For this review, take the finished solid that the model builds, in its own axes (mm). Coordinates: 2 decimals unless noted, no trailing zeros. Loops run counter-clockwise (first coordinate to the right, second up) from the corner with the lowest first, then second, coordinate; pieces in that order, holes last. Notation, with made-up numbers: (42.5, 89) -> (64.5, 89) arc R27 cw to (64.5, 115) -> close; hole circle Ø7 at (71.5, -28.75). An arc over 180 degrees is marked (long way). One line per item, written item: value.
Autodesk Inventor part; units mm, degrees
sketch "Эскиз1" plane through (0, 0, 0) normal (0, 1, 0) x (-1, 0, 0)
  line L0 (105, 10) -> (-105, 10)
  line L1 (-105, -10) -> (105, -10)
  line L2 (105, 10) -> (-105, -10) construction
  line L3 (-105, 10) -> (105, -10) construction
  arc A0 (-105, 10) -> (-105, -10) centre (-105, 0) ccw
  arc A1 (105, -10) -> (105, 10) centre (105, 0) ccw
  line L4 (0, -14) -> (0, 14) construction
  circle A2 centre (105, 0) radius 4
  circle A3 centre (-105, 0) radius 4
  circle A4 centre (0, 0) radius 4
  line L5 (-161, 0) -> (161, 0)
  point P0 (0, 10)
  point P1 (0, -10)
  dimension "d2" = 210
  dimension "d5" = 8
  dimension "d6" = 8
  dimension "d9" = 8
  dimension "d17" = 10
extrude "Выдавливание1" add sketch "Эскиз1" along normal mid plane 4 contours A1 L5 A2 A4 A3 A0 L0 | A1 L1 A0 L5 A3 A4 A2
properties part number "Рельс платформы подъёмника"
1. To check wall thickness, follow probe 1 along X at (y, z) = (-0.75, 0); probe 2 along Z at (x, y) = (105, -0.85); probe 3 along X at (y, z) = (-0.15, -2.75). State the ranges of each line that lie inside material, in increasing order. Write a range as from..to.
Return value:
probe 1: x = -115..-109, -101..-4, 4..101, 109..115
probe 2: z = -10..-4, 4..10
probe 3: x = -114.61..-107.9, -102.1..-2.9, 2.9..102.1, 107.9..114.61
2. Insertion check: pin 1 Ø7 at (x, z) = (-105, 0) entering from -Y; pin 2 Ø2 at (y, z) = (-0.5, 3) entering from +X; pin 3 Ø2 at (y, z) = (-0.5, -3.5) entering from -X. Each pin has a flat end and moves straight along its axis. Give the tip position at first contact, or say it passes through.
Return value:
pin 1: passes through
pin 2: stops at x = 114.8
pin 3: stops at x = -114.68
3. Take a section at A-A, the plane z = 0. Give the boundary of the cut face in (x, y), and give its area (3 significant figures).
Return value:
outline: (-115, -2) -> (-109, -2) -> (-109, 2) -> (-115, 2) -> close; (-101, -2) -> (-4, -2) -> (-4, 2) -> (-101, 2) -> close; (4, -2) -> (101, -2) -> (101, 2) -> (4, 2) -> close; (109, -2) -> (115, -2) -> (115, 2) -> (109, 2) -> close
area: 824 mm2
4. The part is to be moulded in two halves that separate along X. For faces 1 (the flat face through (-1, 0, 10)), 2 (the cylindrical face through (-101, 0, 0)), 3 (the cylindrical face through (-115, 0, 0)), say which applies: pulls with the +X half, pulls with the -X half, needs draft (parallel to the pull), parting line crosses it, or undercut.
Return value:
face 1: needs draft
face 2: undercut
face 3: pulls with the -X half
5. Take a section at B-B, the plane y = 1.25. Give the boundary of the cut face in (x, z).
Return value:
outline: (-105, -10) -> (105, -10) arc R10 ccw to (105, 10) -> (-105, 10) arc R10 ccw to start; hole circle Ø8 at (-105, 0); hole circle Ø8 at (0, 0); hole circle Ø8 at (105, 0)
